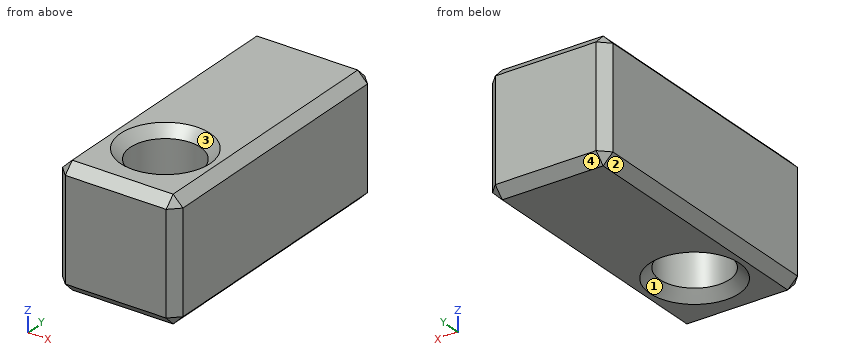
```python
from build123d import *

# Parameters (mm, degrees)
SKETCH1_W           = 21.844
SKETCH1_H           = 21.844
BOSS_EXTRUDE1_DEPTH = 50.8
SKETCH3_R           = 6.35
CUT_EXTRUDE2_DEPTH  = 70.182669358
CHAMFER1_SIZE       = 1.778


with BuildPart() as part:
    # Sketch1 → Boss-Extrude1 (new body)
    with BuildSketch(Plane(origin=(0, 0, 0), x_dir=(1, 0, 0), z_dir=(0, 1, 0))):
        with Locations((-30.652528302, 10.384945755)):
            Rectangle(SKETCH1_W, SKETCH1_H)
    extrude(amount=BOSS_EXTRUDE1_DEPTH)

    # Sketch3 → Cut-Extrude2 (cut, through all)
    with BuildSketch(Plane.XY.offset(0.537054245)):
        with Locations((-30.652528302, 12.7)):
            Circle(SKETCH3_R)
    extrude(amount=-CUT_EXTRUDE2_DEPTH, mode=Mode.SUBTRACT)

    # Chamfer1
    chamfer1_edges = [part.edges().sort_by_distance(p)[0] for p in [
        (-30.652528302, 50.8, 0.537054245),
        (-37.002528302, 12.7, -21.306945755),
        (-37.002528302, 12.7, 0.537054245),
        (-19.730528302, 50.8, -10.384945755),
        (-30.652528302, 50.8, -21.306945755),
        (-19.730528302, 0, -10.384945755),
        (-30.652528302, 0, 0.537054245),
        (-41.574528302, 0, -10.384945755),
        (-30.652528302, 0, -21.306945755),
        (-19.730528302, 25.4, -21.306945755),
        (-19.730528302, 25.4, 0.537054245),
        (-41.574528302, 25.4, 0.537054245),
        (-41.574528302, 25.4, -21.306945755),
        (-41.574528302, 50.8, -10.384945755),
    ]]
    chamfer(chamfer1_edges, length=CHAMFER1_SIZE)


solid = part.part
```
Input: part model. Units: mm. Frame: model coordinates. Face numbers are marked on the shaded views. Coordinates: 2 decimals unless noted, no trailing zeros. Write each loop counter-clockwise with the first axis right and the second up, starting at its lowest first coordinate (ties: lowest second). Pieces come first, ordered by that corner, then holes.
1) Section A-A on z = -18.5. Output: boundary loops of the cut face in (x, y), and give its area (3 significant figures).
2) Material intervals for line 1 along Y through (x, z) = (-30.75, -15.5); line 2 along Y through (x, z) = (-32.25, -17.5); line 3 along X through (y, z) = (12, -19.5), sorted ascending.
3) Mould query, pull axis X, two halves, no side actions, for the marked faces 1, 2, 3 and 4. Classes: pulls with the +X half, pulls with the -X half, needs draft (parallel to the pull), parting line crosses it, or undercut.
4) Pin query (flat end, axial travel): pin 1 Ø1 at (x, y) = (-37.5, 9.5) entering from -Z; pin 2 Ø11.5 at (x, y) = (-30.65, 12.7) entering from -Z. Return the tip coordinate at first contact, or that it passes through.
5) Section B-B on y = 12.7. Output: boundary loops of the cut face in (x, z).
Check result:
1. outline: (-41.57, 1.78) - (-39.8, 0) - (-21.51, 0) - (-19.73, 1.78) - (-19.73, 49.02) - (-21.51, 50.8) - (-39.8, 50.8) - (-41.57, 49.02) - close; hole circle Ø12.7 at (-30.65, 12.7)
1. area: 977 mm2
2. line 1: y = 0 to 6.35, 19.05 to 50.8
2. line 2: y = 0 to 6.55, 18.85 to 50.8
2. line 3: x = -41.57 to -36.96, -24.34 to -19.73
3. face 1: undercut
3. face 2: pulls with the -X half
3. face 3: undercut
3. face 4: needs draft
4. pin 1: stops at z = -21.24
4. pin 2: passes through
5. outline: (-41.57, -19.53) - (-39.8, -21.31) - (-38.78, -21.31) - (-37, -19.53) - (-37, -1.24) - (-38.78, 0.54) - (-39.8, 0.54) - (-41.57, -1.24) - close; (-24.3, -19.53) - (-22.52, -21.31) - (-21.51, -21.31) - (-19.73, -19.53) - (-19.73, -1.24) - (-21.51, 0.54) - (-22.52, 0.54) - (-24.3, -1.24) - close
